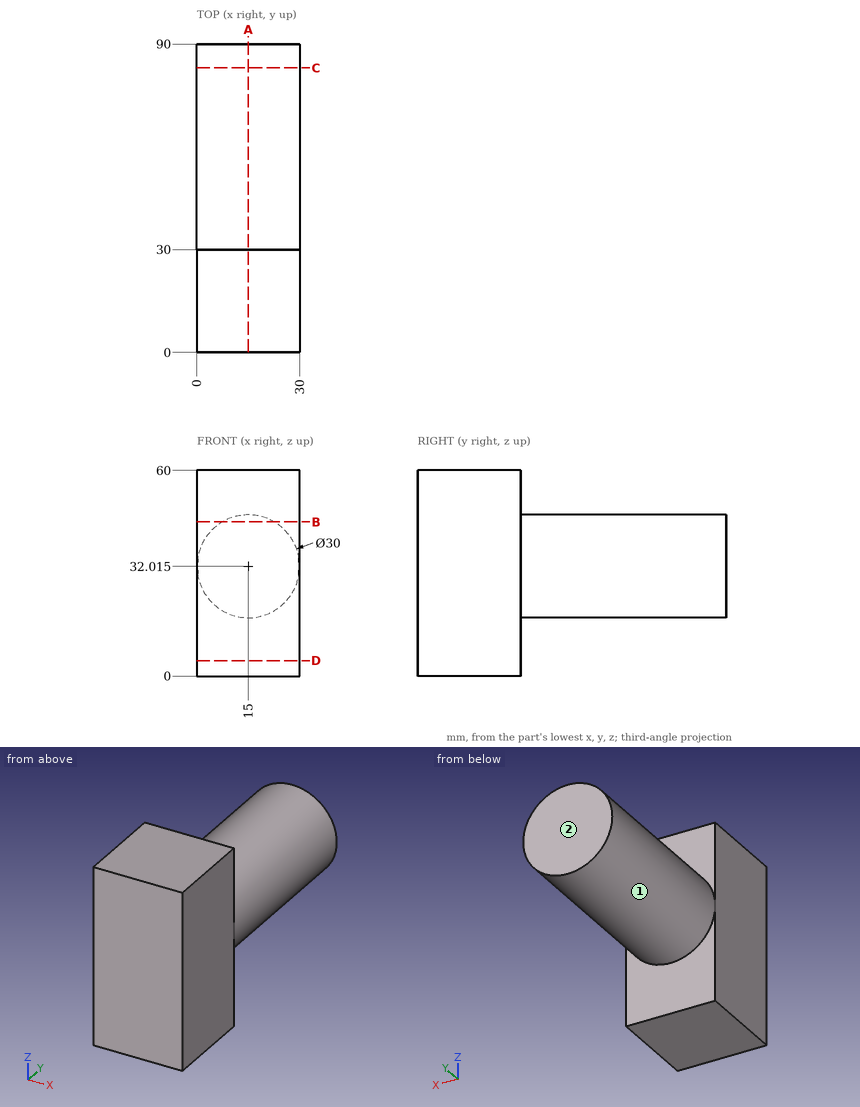
Design review of the part shown in the three views and the two pictorial views. Dimensions are in mm from the part's minimum x, y and z. A direction names the side the tool comes from. Coordinates: 2 decimals unless noted, no trailing zeros. Order: outer loops, then holes, each group sorted by start corner. A loop starts at its lowest first (then second) coordinate and runs counter-clockwise, first axis right, second up.
1) Take a section at D-D, the plane z = 4.5. Give the boundary of the cut face in (x, y), and give its area (3 significant figures).
2) Take a section at A-A, the plane x = 15. Give the boundary of the cut face in (y, z) (1 decimal), and give its area (3 significant figures).
3) Wall thickness on line 1 along Y through (x, z) = (22.75, 7); line 2 along Z through (x, y) = (15.25, 71); line 3 along Z through (x, y) = (11.75, 53.5): over which ranges is each line inside the solid? List them lowest first.
4) Take a section at B-B, the plane z = 45. Give the boundary of the cut face in (x, y), and give its area (3 significant figures).
5) For the marked faces 1 and 2, list the 3-axis set-ups (+Z, -Z, +X, -X, +Y, -Y) from which the entire face can be reached by the end or side of a thin tool; tool diameter is ignored.
6) Take a section at C-C, the plane y = 83. Give the boundary of the cut face in (x, z) (1 decimal).
7) Clearance check with flat-ended pins moving along their axes: pin 1 (3 mm diameter, centred on x = 17.5, y = 59, fed in from +Z); pin 2 (8 mm diameter, centred on x = 22, y = 66.5, fed in from +Z); pin 3 (1 mm diameter, centred on y = 35, z = 29, fed in from -X); pin 4 (10 mm diameter, centred on y = 69, z = 31.5, fed in from -X). State where each tip first meets the part, or that it passes through.
Returned:
1. outline: (0, 0) - (30, 0) - (30, 30) - (0, 30) - close
1. area: 900 mm2
2. outline: (0, 0) - (30, 0) - (30, 17) - (90, 17) - (90, 47) - (30, 47) - (30, 60) - (0, 60) - close
2. area: 3,600 mm2
3. line 1: y = 0 to 30
3. line 2: z = 17.02 to 47.01
3. line 3: z = 17.37 to 46.66
4. outline: (0, 0) - (30, 0) - (30, 30) - (22.51, 30) - (22.51, 90) - (7.49, 90) - (7.49, 30) - (0, 30) - close
4. area: 1,800 mm2
5. face 1: +Y
5. face 2: +Z, -Z, +X, -X, +Y
6. outline: circle Ø30 at (15, 32)
7. pin 1: stops at z = 46.98
7. pin 2: stops at z = 46.71
7. pin 3: stops at x = 0.21
7. pin 4: stops at x = 0
